Read the model definition and answer for the solid it produces. Units are mm, in the model's axes. Face numbers are marked on the shaded views. A direction names the side the tool comes from. Coordinates: 2 decimals unless noted, no trailing zeros. Loops run counter-clockwise (first coordinate to the right, second up) from the corner with the lowest first, then second, coordinate; pieces in that order, holes last. Notation, with made-up numbers: (45.5, 51.5) -> (87.5, 51.5) arc R17 ccw to (87.5, 84.5) -> close; hole circle Ø10 at (-28.5, -8.75). An arc over 180 degrees is marked (long way). Answer as a JSON object with one key per item and string values. Group by question number.
Q1. The part is cut by section B-B on x = 147. Write down the section's boundary in (y, z) (3 decimals).
Q2. This flat-tipped pin is pushed along its axis until it touches: P1, Ø6.5, axis at x = 159, y = 4, coming from the -Z side. Where does it stop, or does it pass through?
Q3. For the marked faces 1, 2 and 3, determine the directions among +Z, -Z, +X, -X, +Y, -Y from which every point of the face is accessible in a straight line to the end or side of a thin tool.
Q4. The part is cut by section C-C on z = 6.5. Write down the section's boundary in (x, y), and give its area (3 significant figures).
Q5. Straight lines are drawn through the part: line 1 along Z through (x, y) = (142, 2.25) (3 decimals); line 2 along Z through (x, y) = (24, 10) (3 decimals). For each, find the intervals that lie inside material, in ascending order. Write a range as [from, to].
Q6. The part is cut by section A-A on y = 6.35. Write down the section's boundary in (x, z) (3 decimals), and give its area (3 significant figures).
from build123d import *

# Parameters (mm, degrees)
SKETCH1_W          = 177.8
SKETCH1_H          = 12.7
BASE_EXTRUDE_DEPTH = 14.605
EXTRUDE1_DEPTH     = 50.8
SKETCH2_R          = 4.064
CUT_EXTRUDE1_DEPTH = 4.175
SKETCH3_R          = 4.064
CUT_EXTRUDE2_DEPTH = 4.175
CHAMFER1_SIZE      = 3.175
CHAMFER2_SIZE      = 3.175


with BuildPart() as part:
    # Sketch1 → Base-Extrude (new body)
    with BuildSketch(Plane.XY):
        with Locations((88.9, 6.35)):
            Rectangle(SKETCH1_W, SKETCH1_H)
    extrude(amount=BASE_EXTRUDE_DEPTH)


with BuildPart() as body_2:
    # Sketch5 → Extrude1 (new body)
    with BuildSketch(Plane(origin=(0, 12.7, 0), x_dir=(-1, 0, 0), z_dir=(0, 1, 0))):
        with BuildLine():
            Line((0, 0), (-47.022766551, 0))
            ThreePointArc((-47.022766551, 0), (-50.789601569, 0.139848461), (-54.535696978, 0.55862386))
            Line((-54.535696978, 0.55862386), (-123.733861174, 10.906290131))
            ThreePointArc((-123.733861174, 10.906290131), (-127.245825619, 11.298892068), (-130.777233449, 11.43))
            Line((-130.777233449, 11.43), (-177.8, 11.43))
            Line((-177.8, 11.43), (-177.8, 14.605))
            Line((-177.8, 14.605), (-130.777233449, 14.605))
            ThreePointArc((-130.777233449, 14.605), (-127.010398431, 14.465151539), (-123.264303022, 14.04637614))
            Line((-123.264303022, 14.04637614), (-54.066138826, 3.698709869))
            ThreePointArc((-54.066138826, 3.698709869), (-50.554174381, 3.306107932), (-47.022766551, 3.175))
            Line((-47.022766551, 3.175), (0, 3.175))
            Line((0, 3.175), (0, 0))
        make_face()
    extrude(amount=-EXTRUDE1_DEPTH)


with BuildPart() as part_1:
    add(part.part)

    # Combine1: intersect body 2
    add(body_2.part, mode=Mode.INTERSECT)

    # Sketch2 → Cut-Extrude1 (cut, through all)
    with BuildSketch(Plane.XY.offset(3.175)):
        with Locations((8.128, 6.35)):
            Circle(SKETCH2_R)
    extrude(amount=-CUT_EXTRUDE1_DEPTH, mode=Mode.SUBTRACT)

    # Sketch3 → Cut-Extrude2 (cut, through all)
    with BuildSketch(Plane(origin=(185.269572221, -0.228654981, 11.43), x_dir=(1, 0, 0), z_dir=(0, 0, 1))):
        with Locations((-15.597572221, 6.578654981)):
            Circle(SKETCH3_R)
    extrude(amount=CUT_EXTRUDE2_DEPTH, mode=Mode.SUBTRACT)

    # Chamfer1
    chamfer1_edges = [part_1.edges().sort_by_distance(p)[0] for p in [
        (177.8, 0, 13.0175),
        (177.8, 12.7, 13.0175),
    ]]
    chamfer(chamfer1_edges, length=CHAMFER1_SIZE)

    # Chamfer2
    chamfer2_edges = [part_1.edges().sort_by_distance(p)[0] for p in [
        (0, 12.7, 1.5875),
        (0, 0, 1.5875),
    ]]
    chamfer(chamfer2_edges, length=CHAMFER2_SIZE)


solid = part_1.part
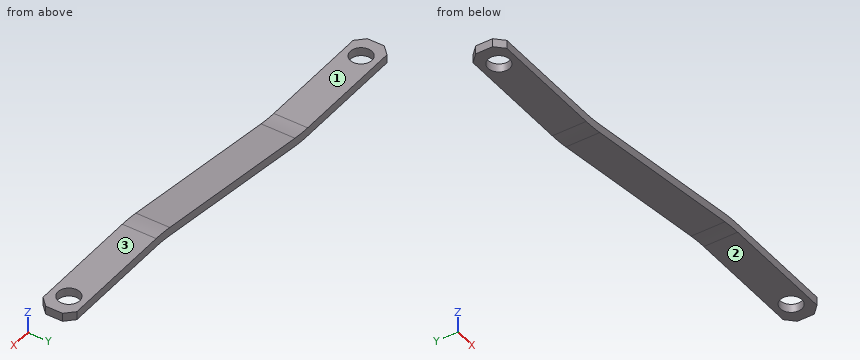
Final values:
{
 "1": {"outline": "(0, 11.43) -> (12.7, 11.43) -> (12.7, 14.605) -> (0, 14.605) -> close"},
 "2": {"P1": "stops at z = 11.43"},
 "3": {"face 1": "+Z, -X, +Y, -Y", "face 2": "-Z, +X, +Y, -Y", "face 3": "+Z, +X, -X, +Y, -Y"},
 "4": {"outline": "(72.8, 0) -> (94.27, 0) -> (94.27, 12.7) -> (72.8, 12.7) -> close", "area": "273 mm2"},
 "5": {"line 1": "z = [11.43, 14.605]", "line 2": "z = [0, 3.175]"},
 "6": {"outline": "(0, 0) -> (4.064, 0) -> (4.064, 3.175) -> (0, 3.175) -> close; (12.192, 0) -> (47.023, 0) arc R50.8 ccw to (54.536, 0.559) -> (123.734, 10.906) arc R47.625 cw to (130.777, 11.43) -> (165.608, 11.43) -> (165.608, 14.605) -> (130.777, 14.605) arc R50.8 ccw to (123.264, 14.046) -> (54.066, 3.699) arc R47.625 cw to (47.023, 3.175) -> (12.192, 3.175) -> close; (173.736, 11.43) -> (177.8, 11.43) -> (177.8, 14.605) -> (173.736, 14.605) -> close", "area": "516 mm2"}
}
